from build123d import *

# Parameters (mm, degrees)
BOSS_EXTRUDE1_START = 2.5
SKETCH1_R           = 144
BOSS_EXTRUDE1_DEPTH = 10
SKETCH2_R           = 80.5
CUT_EXTRUDE1_DEPTH  = 1
SKETCH3_R           = 65.5
CUT_EXTRUDE2_DEPTH  = 204.845529752
SKETCH4_R           = 74.125
SKETCH4_R_2         = 65.5
BOSS_EXTRUDE3_DEPTH = 36.33
BOSS_EXTRUDE4_START = -7.2
SKETCH5_R           = 74.125
BOSS_EXTRUDE4_DEPTH = 7.2
SKETCH6_R           = 34
CUT_EXTRUDE3_DEPTH  = 17.2
SKETCH7_R           = 144
SKETCH7_R_2         = 80.5
BOSS_EXTRUDE5_DEPTH = 15
CHAMFER2_SIZE       = 4
SKETCH10_R          = 7.65
CUT_EXTRUDE4_DEPTH  = 207.437566591
CIRPATTERN2_COUNT   = 5
CHAMFER3_SIZE       = 2
CUT_EXTRUDE6_DEPTH  = 2


with BuildPart() as part:
    # Sketch1 → Boss-Extrude1 (new body)
    with BuildSketch(Plane.XY.offset(BOSS_EXTRUDE1_START)):
        Circle(SKETCH1_R)
    extrude(amount=BOSS_EXTRUDE1_DEPTH)

    # Sketch2 → Cut-Extrude1 (cut)
    with BuildSketch(Plane.XY.offset(12.5)):
        Circle(SKETCH2_R)
    extrude(amount=-CUT_EXTRUDE1_DEPTH, mode=Mode.SUBTRACT)

    # Sketch3 → Cut-Extrude2 (cut, through all)
    with BuildSketch(Plane.XY.offset(11.5)):
        Circle(SKETCH3_R)
    extrude(amount=-CUT_EXTRUDE2_DEPTH, mode=Mode.SUBTRACT)

    # Sketch4 → Boss-Extrude3 (add)
    with BuildSketch(Plane(origin=(0, 0, 2.5), x_dir=(-1, 0, 0), z_dir=(0, 0, -1))):
        with Locations(Location((0, 0, 0), (0, 0, 180))):
            Circle(SKETCH4_R)
        with Locations(Location((0, 0, 0), (0, 0, 180))):
            Circle(SKETCH4_R_2, mode=Mode.SUBTRACT)
    extrude(amount=BOSS_EXTRUDE3_DEPTH)

    # Sketch5 → Boss-Extrude4 (add)
    with BuildSketch(Plane(origin=(0, 0, -33.83), x_dir=(-1, 0, 0), z_dir=(0, 0, -1)).offset(BOSS_EXTRUDE4_START)):
        with Locations(Location((0, 0, 0), (0, 0, 180))):
            Circle(SKETCH5_R)
    extrude(amount=BOSS_EXTRUDE4_DEPTH)

    # Sketch6 → Cut-Extrude3 (cut)
    with BuildSketch(Plane.XY.offset(-26.63)):
        Circle(SKETCH6_R)
    extrude(amount=-CUT_EXTRUDE3_DEPTH, mode=Mode.SUBTRACT)

    # Sketch7 → Boss-Extrude5 (add)
    with BuildSketch(Plane(origin=(0, 0, 2.5), x_dir=(-1, 0, 0), z_dir=(0, 0, -1))):
        Circle(SKETCH7_R)
        with Locations(Location((0, 0, 0), (0, 0, 180))):
            Circle(SKETCH7_R_2, mode=Mode.SUBTRACT)
    extrude(amount=BOSS_EXTRUDE5_DEPTH)

    # Chamfer2
    chamfer2_edges = [part.edges().sort_by_distance(p)[0] for p in [
        (-34, 0, -33.83),
    ]]
    chamfer(chamfer2_edges, length=CHAMFER2_SIZE)

    # Sketch10 → Cut-Extrude4 (cut, through all)
    with BuildSketch(Plane.XY):
        with Locations((56, 0)):
            Circle(SKETCH10_R)
    cut_extrude4 = extrude(amount=-CUT_EXTRUDE4_DEPTH, mode=Mode.SUBTRACT)

    # CirPattern2: Cut-Extrude4 ×5 about axis
    cirpattern2_axis = Axis((0, 0, 0), (0, 0, 1))
    for i in range(1, CIRPATTERN2_COUNT):
        add(cut_extrude4.rotate(cirpattern2_axis, i * 360 / CIRPATTERN2_COUNT), mode=Mode.SUBTRACT)

    # Chamfer3
    chamfer3_edges = [part.edges().sort_by_distance(p)[0] for p in [
        (-74.125, 0, -33.83),
    ]]
    chamfer(chamfer3_edges, length=CHAMFER3_SIZE)

    # Sketch12 → Cut-Extrude6 (cut)
    with BuildSketch(Plane(origin=(0, 0, -12.5), x_dir=(-1, 0, 0), z_dir=(0, 0, -1))):
        Polygon((-43.036764008, -72.137625021), (-71.215597585, -119.370593785), (-67.780472584, -121.4199635), (-39.601639007, -74.186994736), align=None)
        Polygon((-82.692946132, -15.293026515), (-137.190383486, -22.711201621), (-137.72988713, -18.747751632), (-83.232449776, -11.329576526), align=None)
        Polygon((-63.514778191, 55.116902592), (-103.293137449, 93.099558302), (-100.530762488, 95.992529884), (-60.75240323, 58.009874175), align=None)
        Polygon((3.491313194, 84.022679868), (8.385947883, 138.804451939), (12.370076761, 138.448478507), (7.475442071, 83.666706436), align=None)
        Polygon((67.868374533, 49.657665453), (113.750243417, 79.986762171), (115.955995905, 76.64989898), (70.074127022, 46.320802261), align=None)
        Polygon((81.139165587, -22.10058388), (133.458285575, -39.062590944), (132.224685062, -42.867617853), (79.905565073, -25.905610789), align=None)
        Polygon((33.310510016, -77.216642782), (52.669516643, -128.697016347), (48.925489474, -130.104944102), (29.566482848, -78.624570536), align=None)
    extrude(amount=-CUT_EXTRUDE6_DEPTH, mode=Mode.SUBTRACT)


solid = part.part
The model under review builds one solid part; all positions refer to its coordinate system, in mm. A direction names the side the tool comes from. Coordinates: 2 decimals unless noted, no trailing zeros. Order: outer loops, then holes, each group sorted by start corner. A loop starts at its lowest first (then second) coordinate and runs counter-clockwise, first axis right, second up. Notation, with made-up numbers: (62.5, -24.5) -> (109.5, -24.5) arc R24 ccw to (109.5, -2.5) -> close; hole circle Ø4 at (-28, 18). An arc over 180 degrees is marked (long way). Answer in a Markdown table with one row per item.
(1) The part is to be moulded in two halves that separate along X. For faces 1 (the flat face through (53.888, -98.134, -11.514)), 2 (the flat face through (31, 31, -33.83)), 3 (the conical face through (68.914, -21.702, -33.705)), 4 (the cylindrical face through (-52.744, -34.699, -30.18)), say which applies: +X half, -X half, draft (parallel to the pull), parting line (faces both ways), or undercut.
Answers:
| item | result |
|---|---|
| face 1 | undercut |
| face 2 | draft |
| face 3 | parting line |
| face 4 | undercut |
(2) Consider section D-D (x = 113.5). Write out the cut boundary in (y, z), plus the area to 3 significant figures.
Answers:
| item | result |
|---|---|
| outline | (-88.62, -12.5) -> (-19.49, -12.5) -> (-19.49, -10.5) -> (-15.45, -10.5) -> (-15.45, -12.5) -> (88.62, -12.5) -> (88.62, 12.5) -> (-88.62, 12.5) -> close |
| area | 4,420 mm² |
(3) Insertion check: pin 1 (7 mm diameter, centred on x = -42, y = -93.5, fed in from -Z); pin 2 (2 mm diameter, centred on x = -2, z = -24.5, fed in from -Y); pin 3 (20 mm diameter, centred on x = 17.3, y = 53.26, fed in from +Z). Each pin has a flat end and moves straight along its axis. Give the tip position at first contact, or say it passes through.
Answers:
| item | result |
|---|---|
| pin 1 | z = -12.5 |
| pin 2 | y = -74.12 |
| pin 3 | z = 11.5 |
(4) Machinability: for faces 5 (the cylindrical face through (-44.17, 40.48, -30.18)), 6 (the flat face through (56.929, -95.423, -11.514)), which of the approach directions +Z, -Z, +X, -X, +Y, -Y give a long, thin tool a straight path to every point of the face, cutting with its end or side? Answer none if there is none.
Answers:
| item | result |
|---|---|
| face 5 | +Z, -Z |
| face 6 | -Z |
(5) Consider section A-A (x = 0). Write out the cut boundary in (y, z) (3 decimals), plus the area to 3 significant figures.
Answers:
| item | result |
|---|---|
| outline | (-144, -12.5) -> (-80.5, -12.5) -> (-80.5, 2.5) -> (-74.125, 2.5) -> (-74.125, -31.83) -> (-72.125, -33.83) -> (-38, -33.83) -> (-34, -29.83) -> (-34, -26.63) -> (-65.5, -26.63) -> (-65.5, 11.5) -> (-80.5, 11.5) -> (-80.5, 12.5) -> (-144, 12.5) -> close; (34, -29.83) -> (38, -33.83) -> (72.125, -33.83) -> (74.125, -31.83) -> (74.125, 2.5) -> (80.5, 2.5) -> (80.5, -12.5) -> (144, -12.5) -> (144, 12.5) -> (80.5, 12.5) -> (80.5, 11.5) -> (65.5, 11.5) -> (65.5, -26.63) -> (34, -26.63) -> close |
| area | 4,510 mm² |
(6) Consider section C-C (z = 6). Write out the cut boundary in (x, y), plus the area to 3 significant figures.
Answers:
| item | result |
|---|---|
| outline | circle Ø288 at (0, 0); hole circle Ø131 at (0, 0) |
| area | 51,700 mm² |
(7) Wall thickness on line 1 along Y through (x, z) = (0, -3.5) (3 decimals); line 2 along X through (y, z) = (-1, -8.5); line 3 along X through (y, z) = (41, -1): over which ranges is each line inside the solid? List them lowest first.
Answers:
| item | result |
|---|---|
| line 1 | -144 to -80.5, -74.125 to -65.5, 65.5 to 74.125, 80.5 to 144 |
| line 2 | -144 to -80.49, -74.12 to -65.49, 65.49 to 74.12, 80.49 to 144 |
| line 3 | -138.04 to -69.28, -61.75 to -51.08, 51.08 to 61.75, 69.28 to 138.04 |
(8) Consider section B-B (y = 0). State how many separate pieces and enclosed holes the cut face has, plus the area to 3 significant figures.
Answers:
| item | result |
|---|---|
| separate pieces | 3 |
| enclosed holes | 0 |
| area | 4,400 mm² |
